Could you check a few things on this model? Use its own coordinates, in mm. A direction names the side the tool comes from. Coordinates: 2 decimals unless noted, no trailing zeros.
from build123d import *

# Parameters (mm, degrees)
SKETCH1_W               = 914.4
SKETCH1_H               = 9.525
BOSS_EXTRUDE1_DEPTH     = 63.5
SKETCH2_W               = 25.4
SKETCH2_H               = 63.5
CUT_EXTRUDE1_DEPTH      = 6.35
F_1_4_CLEARANCE_HOLE1_D = 6.7564
F_1_4_CLEARANCE_HOLE2_D = 6.7564
LPATTERN1_COUNT         = 3
LPATTERN1_PITCH         = 15.875
MIRROR1_COPY_1_D        = 6.7564


with BuildPart() as part:
    # Sketch1 → Boss-Extrude1 (new body)
    with BuildSketch(Plane(origin=(0, 0, 0), x_dir=(1, 0, 0), z_dir=(0, 1, 0))):
        with Locations((0, 4.7625)):
            Rectangle(SKETCH1_W, SKETCH1_H)
    extrude(amount=BOSS_EXTRUDE1_DEPTH)

    # Sketch2 → Cut-Extrude1 (cut)
    with BuildSketch(Plane(origin=(0, 0, -9.525), x_dir=(-1, 0, 0), z_dir=(0, 0, -1))):
        with Locations((-425.45, 31.75)):
            Rectangle(SKETCH2_W, SKETCH2_H)
    cut_extrude1 = extrude(amount=-CUT_EXTRUDE1_DEPTH, mode=Mode.SUBTRACT)

    # 1/4 Clearance Hole1 (through all)
    with Locations(Plane.XY):
        with Locations((425.45, 47.625)):
            f_1_4_clearance_hole1 = Hole(F_1_4_CLEARANCE_HOLE1_D / 2)

    # 1/4 Clearance Hole2 (through all)
    with Locations(Plane.XY):
        with Locations((-95.25, 41.275), (-95.25, 20.6375), (95.25, 41.275), (95.25, 20.6375)):
            Hole(F_1_4_CLEARANCE_HOLE2_D / 2)

    # LPattern1: 1/4 Clearance Hole1 ×3, 1 skipped
    with Locations(*[(0, -i * LPATTERN1_PITCH, 0) for i in range(1, LPATTERN1_COUNT) if i not in (1,)]):
        add(f_1_4_clearance_hole1, mode=Mode.SUBTRACT)

    # Mirror1: Cut-Extrude1, 1/4 Clearance Hole1 across plane
    add(cut_extrude1.mirror(Plane(origin=(0, 0, 0), x_dir=(0, 0, 1), z_dir=(1, 0, 0))), mode=Mode.SUBTRACT)
    add(f_1_4_clearance_hole1.mirror(Plane(origin=(0, 0, 0), x_dir=(0, 0, 1), z_dir=(1, 0, 0))), mode=Mode.SUBTRACT)

    # Mirror1 copy 1 (through all)
    with Locations(Plane(origin=(0, -31.75, 0), x_dir=(-1, 0, 0), z_dir=(0, 0, 1))):
        with Locations((425.45, -47.625)):
            Hole(MIRROR1_COPY_1_D / 2)


solid = part.part
(1) Which directions (+Z, -Z, +X, -X, +Y, -Y) give clear straight access to the entire face, cutting with the end or side of a thin tool? Please do faces 1 (the face through (-426, 32, -3.175)), 2 (the face through (-448, 31, -9.525)).
Answers:
face 1: -Z, +Y, -Y
face 2: -Z, +X, -X, +Y, -Y
(2) I need wall thicknesses on probe 1 along X at (y, z) = (53, -7); probe 2 along Y at (x, z) = (-425.45, -2.35); probe 3 along X at (y, z) = (19, -4). Which ranges of each line are inside material? Lowest first, please.
Answers:
probe 1: x = -457.2 to -438.15, -412.75 to 412.75, 438.15 to 457.2
probe 2: y = 0 to 12.5, 19.25 to 44.25, 51 to 63.5
probe 3: x = -457.2 to -438.15, -412.75 to -98.2, -92.3 to 92.3, 98.2 to 412.75, 438.15 to 457.2
(3) Imagine slicing it at A-A, the plane z = -5.5. State how many separate pieces and enclosed holes the cut face has, and give its area (3 significant figures).
Answers:
separate pieces: 3
enclosed holes: 4
area: 54,700 mm2
(4) For pin 1 (5.5 mm diameter, centred on x = 425.45, y = 15.875, fed in from +Z); pin 2 (11 mm diameter, centred on x = 425.45, y = 47.625, fed in from -Z) (3 decimals), each with a flat end and sliding along its axis, tell me the tip position at first contact or that it passes through.
Answers:
pin 1: passes through
pin 2: stops at z = -3.175
